Can you work these out from the drawing? Everything is in mm from the part's minimum corner. Round coordinates to 2 decimals unless told otherwise and drop trailing zeros. Loops run counter-clockwise (first coordinate to the right, second up) from the corner with the lowest first, then second, coordinate; pieces in that order, holes last. Notation, with made-up numbers: M -35,50.25 L 6,50.25 A13 cw 6,56.25 Z; hole C -39.75,48 d9. An arc over 180 degrees is marked long. Return JSON: item names as keys, results as strings. Group by question number.
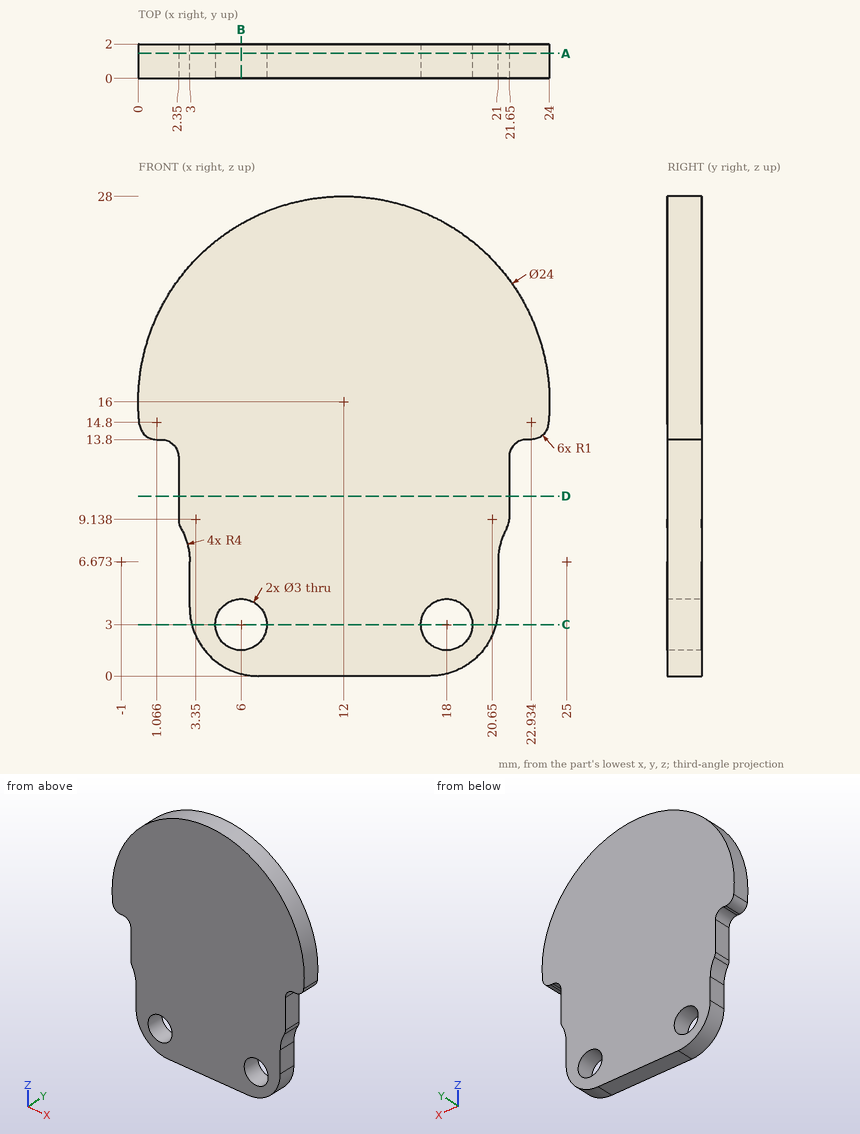
1. If we section it at D-D, the plane z = 10.5: Please give me the cut outline in (x, y).
2. I need wall thicknesses on probe 1 along X at (y, z) = (1.4, 3); probe 2 along X at (y, z) = (1.8, 2) (1 decimal); probe 3 along Z at (x, y) = (6, 1.15). Which ranges of each line are inside material? Lowest first, please.
3. If we section it at A-A, the plane y = 1.45: Give the number of separate pieces and of enclosed holes in the cut face.
4. If we section it at C-C, the plane z = 3: Please give me the cut outline in (x, y), then the cut area to 3 significant figures.
5. I'm going to push flat-ended pins straight in: pin 1 Ø1.5 at (x, z) = (6.5, 3) entering from -Y; pin 2 Ø1 at (y, z) = (1, 10) entering from -X; pin 3 Ø0.6 at (y, z) = (1, 11.5) entering from +X. Where does each tip first touch, or does it pass through?
6. If we section it at B-B, the plane x = 6: Please give me the cut outline in (y, z).
Geometry results:
{
 "1": {"outline": "M 2.35,0 L 21.65,0 L 21.65,2 L 2.35,2 Z"},
 "2": {"probe 1": "3.13 to 4.5, 7.5 to 16.5, 19.5 to 20.87", "probe 2": "3.5 to 4.9, 7.1 to 16.9, 19.1 to 20.5", "probe 3": "0.13 to 1.5, 4.5 to 26.39"},
 "3": {"separate pieces": "1", "enclosed holes": "2"},
 "4": {"outline": "M 3.13,0 L 4.5,0 L 4.5,2 L 3.13,2 Z; M 7.5,0 L 16.5,0 L 16.5,2 L 7.5,2 Z; M 19.5,0 L 20.87,0 L 20.87,2 L 19.5,2 Z", "area": "23.5 mm^2"},
 "5": {"pin 1": "through", "pin 2": "x = 2.35", "pin 3": "x = 21.65"},
 "6": {"outline": "M 0,0.13 L 2,0.13 L 2,1.5 L 0,1.5 Z; M 0,4.5 L 2,4.5 L 2,26.39 L 0,26.39 Z"}
}
